CAD build for the part. Positions are in the model's coordinates, mm. A direction names the side the tool comes from. Round coordinates to 2 decimals unless told otherwise and drop trailing zeros. Write each loop counter-clockwise with the first axis right and the second up, starting at its lowest first coordinate (ties: lowest second). Pieces come first, ordered by that corner, then holes. Notation, with made-up numbers: (-23, 14.5) -> (-5, 14.5) arc R9 ccw to (-5, 21.5) -> close; hole circle Ø7 at (80, 34.5). An arc over 180 degrees is marked (long way). Answer in a Markdown table with one row per item. Add a question column.
```python
from build123d import *

# Parameters (mm, degrees)
F0_R            = 14.8770011714
F0_R_2          = 3.048
F1_DEPTH        = 3.175
F3_DEPTH        = 3.175
F3_COPIES_COUNT = 30


# Not quite as in the source:
# - a pattern or mirror of a feature is missing from the dataset's text; its kind, count and spacing are read off the source's solid


with BuildPart() as f1:
    # F0 (on Top) → F1 (new body)
    with BuildSketch(Plane.XY):
        Circle(F0_R)
        Circle(F0_R_2, mode=Mode.SUBTRACT)
    extrude(amount=F1_DEPTH)

    # F2 (on face) → F3 (cut, through all)
    with BuildSketch(Plane.XY.offset(3.175)):
        with BuildLine():
            Line((0.2742033495, 12.8709727929), (1.1020387684, 14.8361273386))
            ThreePointArc((1.1020387684, 14.8361273386), (0, 14.8770011714), (-1.1020387684, 14.8361273386))
            Line((-1.1020387684, 14.8361273386), (-0.2742033495, 12.8709727929))
            ThreePointArc((-0.2742033495, 12.8709727929), (0, 12.6889428931), (0.2742033495, 12.8709727929))
        make_face()
    f3 = extrude(amount=-F3_DEPTH, mode=Mode.SUBTRACT)

    # F3_copies: F3 ×30 about axis
    f3_copies_axis = Axis((0, 0, 0), (0, 0, 1))
    for i in range(1, F3_COPIES_COUNT):
        add(f3.rotate(f3_copies_axis, i * 360 / F3_COPIES_COUNT), mode=Mode.SUBTRACT)


solid = f1.part
```
Item 1: Pin check, flat tips, straight feed: pin 1 (1.5 mm diameter, centred on x = 9.5, y = 0, fed in from -Z); pin 2 (1.5 mm diameter, centred on x = -11.5, z = 1.5, fed in from -Y); pin 3 (5.5 mm diameter, centred on x = 0, y = 0, fed in from -Z); pin 4 (1.5 mm diameter, centred on y = 1, z = 1, fed in from +X). Stop position of each tip, or through.
Item 2: Saw through at B-B on x = -8.25. Give the cut face in (y, z) (3 decimals).
Item 3: Two-plate mould, pull along Y, no slides. Class faces 1 (the flat face through (3.56, -13.42, 1.61)), 2 (the flat face through (10.742, 8.754, 1.61)), 3 (the flat face through (-3.56, 13.42, 1.61)): +Y half, -Y half, draft (parallel to the pull), parting line (faces both ways), or undercut.
Item 4: Tool access for faces 4 (the flat face through (-13.72, -2.14, 1.61)), 5 (the flat face through (-10.742, -8.754, 1.61)), 6 (the flat face through (0.682, 13.84, 1.61)), 7 (the flat face through (13.86, -0.76, 1.61)): list every direction of +Z, -Z, +X, -X, +Y, -Y with a clear straight run to the whole face (end or side of a thin tool).
Item 5: Saw through at A-A on y = 0. Give the cut face in (x, z) (3 decimals).
Item 6: Drill centre lines: probe 1 along Y at (x, z) = (0, 1.75); probe 2 along X at (y, z) = (13.5, 3); probe 3 along Y at (x, z) = (-13, 0.4). Where is each one in solid material? Low to high.
Recorded:
| question | item | result |
|---|---|---|
| 1 | pin 1 | z = 0 |
| 1 | pin 2 | y = -9.11 |
| 1 | pin 3 | through |
| 1 | pin 4 | x = 14.87 |
| 2 | outline | (-10.531, 0) -> (10.531, 0) -> (10.531, 3.175) -> (-10.531, 3.175) -> close |
| 3 | face 1 | -Y half |
| 3 | face 2 | undercut |
| 3 | face 3 | +Y half |
| 4 | face 4 | +Z, -Z, -X |
| 4 | face 5 | +Z, -Z |
| 4 | face 6 | +Z, -Z, +Y |
| 4 | face 7 | +Z, -Z, +X |
| 5 | outline | (-14.877, 0) -> (-3.048, 0) -> (-3.048, 3.175) -> (-14.877, 3.175) -> close; (3.048, 0) -> (14.877, 0) -> (14.877, 3.175) -> (3.048, 3.175) -> close |
| 6 | probe 1 | -12.69 to -3.05, 3.05 to 12.69 |
| 6 | probe 2 | -5.02 to -3.62, -2.24 to -0.54, 0.54 to 2.24, 3.62 to 5.02 |
| 6 | probe 3 | -6.41 to -4.97, -3.66 to -1.74, -1.02 to 1.02, 1.74 to 3.66, 4.97 to 6.41 |
